from build123d import *

# Parameters (mm, degrees)
EXTRUDE_2_DEPTH     = 127
EXTRUDE_3_DEPTH     = 28.575
EXTRUDE_6_DEPTH     = 31.75
SKETCH_5_R          = 25.4
CUT_EXTRUDE_4_DEPTH = 31.75
SKETCH_6_W          = 76.2
SKETCH_6_H          = 3.175
CUT_EXTRUDE_5_DEPTH = 136.525


with BuildPart() as part:
    # 草图1 → 凸台-拉伸2 (new body)
    with BuildSketch(Plane(origin=(0, 0, 0), x_dir=(0, 0, -1), z_dir=(1, 0, 0))):
        with BuildLine():
            Line((0, 0), (107.95, 0))
            Line((107.95, 0), (107.95, 75.565))
            Line((107.95, 75.565), (76.2, 75.565))
            Line((76.2, 75.565), (76.2, 34.925))
            ThreePointArc((76.2, 34.925), (72.480256121, 25.944743879), (63.5, 22.225))
            Line((63.5, 22.225), (0, 22.225))
            Line((0, 22.225), (0, 0))
        make_face()
    extrude(amount=-EXTRUDE_2_DEPTH)

    # 草图2 → 凸台-拉伸3 (add)
    with BuildSketch(Plane.XY):
        Polygon((0, 0), (0, 31.75), (-25.4, 31.75), (-25.4, 22.225), (-101.6, 22.225), (-101.6, 31.75), (-127, 31.75), (-127, 0), align=None)
    extrude(amount=EXTRUDE_3_DEPTH)

    # 草图3 → 凸台-拉伸6 (add)
    with BuildSketch(Plane(origin=(0, 0, -107.95), x_dir=(-1, 0, 0), z_dir=(0, 0, -1))):
        with BuildLine():
            Line((0, 75.565), (0, 139.065))
            ThreePointArc((0, 139.065), (3.719743879, 148.045256121), (12.7, 151.765))
            Line((12.7, 151.765), (114.3, 151.765))
            ThreePointArc((114.3, 151.765), (123.280256121, 148.045256121), (127, 139.065))
            Line((127, 139.065), (127, 75.565))
            Line((127, 75.565), (0, 75.565))
        make_face()
    extrude(amount=-EXTRUDE_6_DEPTH)

    # 草图5 → 切除-拉伸4 (cut)
    with BuildSketch(Plane(origin=(0, 0, -107.95), x_dir=(-1, 0, 0), z_dir=(0, 0, -1))):
        with Locations((63.5, 100.965)):
            Circle(SKETCH_5_R)
    extrude(amount=-CUT_EXTRUDE_4_DEPTH, mode=Mode.SUBTRACT)

    # 草图6 → 切除-拉伸5 (cut)
    with BuildSketch(Plane.XY.offset(28.575)):
        with Locations((-63.5, 1.5875)):
            Rectangle(SKETCH_6_W, SKETCH_6_H)
    extrude(amount=-CUT_EXTRUDE_5_DEPTH, mode=Mode.SUBTRACT)


solid = part.part
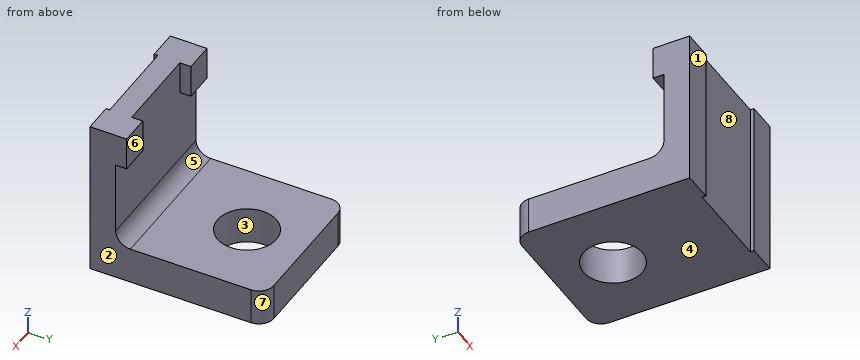
Work out the finished part from the listing and answer in its coordinate system (mm). Face numbers are marked on the shaded views. A direction names the side the tool comes from. Coordinates: 2 decimals unless noted, no trailing zeros. Loops run counter-clockwise (first coordinate to the right, second up) from the corner with the lowest first, then second, coordinate; pieces in that order, holes last. Notation, with made-up numbers: (8, 89) -> (21, 89) arc R14 cw to (21, 104) -> close; hole circle Ø7 at (10.5, 32.5). An arc over 180 degrees is marked (long way). Write each question's results on one line, items separated by ' | '. Start each with the question number.
1) Consider line 1 along Y through (x, z) = (-63.5, -91.5) (3 decimals); line 2 along Z through (x, y) = (-92, 92.5); line 3 along Y through (x, z) = (-101.5, -79) (3 decimals). Determine where each line is inside the solid, lowest interval first.
2) Find section C-C on y = 104.5. Determine the outline of the cut face in (x, z).
3) Flat-ended cylindrical pins translate along their axes: P1, Ø10, axis at x = -26.5, z = -72, coming from the -Y side; P2, Ø20.5, axis at x = -109.5, z = 21, coming from the +Y side; P3, Ø8, axis at x = -82, z = -24.5, coming from the +Y side (3 decimals); P4, Ø10, axis at x = -49.5, z = -20, coming from the -Y side (3 decimals). Find the tip coordinate at first contact, or state that the pin passes through.
4) Find section D-D on x = -83.5. Determine the outline of the cut face in (y, z) (3 decimals).
5) For the marked faces 4, 5, 6, 7 and 8, determine the directions among +Z, -Z, +X, -X, +Y, -Y from which every point of the face is accessible in a straight line to the end or side of a thin tool.
6) The mould has two halves that part along X. Classify the marked faces 1, 2 and 3: pulls with the +X half, pulls with the -X half, needs draft (parallel to the pull), parting line crosses it, or undercut.
7) Find section B-B on z = -19. Determine the outline of the cut face in (x, y) (3 decimals), then the cut area to 3 significant figures.
8) Find section A-A on x = -63.5. Determine the outline of the cut face in (y, z) (3 decimals).
Response values:
1) line 1: y = 3.175 to 75.565, 126.365 to 151.765 | line 2: z = -107.95 to -76.2 | line 3: y = 3.175 to 151.765
2) outline: (-127, -107.95) -> (-88.65, -107.95) -> (-88.65, -76.2) -> (-127, -76.2) -> close; (-38.35, -107.95) -> (0, -107.95) -> (0, -76.2) -> (-38.35, -76.2) -> close
3) P1: stops at y = 0 | P2: stops at y = 31.75 | P3: stops at y = 22.225 | P4: stops at y = 3.175
4) outline: (3.175, -107.95) -> (85.307, -107.95) -> (85.307, -76.2) -> (34.925, -76.2) arc R12.7 cw to (22.225, -63.5) -> (22.225, 28.575) -> (3.175, 28.575) -> close; (116.623, -107.95) -> (151.765, -107.95) -> (151.765, -76.2) -> (116.623, -76.2) -> close
5) face 4: -Z, +X, -X, +Y, -Y | face 5: +X, -X, +Y | face 6: +Z, +X, -X, +Y | face 7: +Z, -Z, +X, +Y | face 8: +Z, -Z, -Y
6) face 1: needs draft | face 2: pulls with the +X half | face 3: undercut
7) outline: (-127, 0) -> (-101.6, 0) -> (-101.6, 3.175) -> (-25.4, 3.175) -> (-25.4, 0) -> (0, 0) -> (0, 22.225) -> (-127, 22.225) -> close | area: 2,580 mm^2
8) outline: (3.175, -107.95) -> (75.565, -107.95) -> (75.565, -76.2) -> (34.925, -76.2) arc R12.7 cw to (22.225, -63.5) -> (22.225, 28.575) -> (3.175, 28.575) -> close; (126.365, -107.95) -> (151.765, -107.95) -> (151.765, -76.2) -> (126.365, -76.2) -> close
